```python
from build123d import *

# Parameters (mm, degrees)
SKETCH_R  = 1.25
PAD_DEPTH = 10
FILLET_R  = 1


with BuildPart() as part:
    # Sketch → Pad (new body)
    with BuildSketch(Plane.XY):
        Polygon((-7.5, 7.5), (-1.7, 7.5), (-1.7, 6.4), (-2.85, 6.4), (-2.85, 3.8), (-1.7, 2.802683), (1.7, 2.802683), (2.85, 3.8), (2.85, 6.4), (1.7, 6.4), (1.7, 7.5), (7.5, 7.5), (7.5, 1.7), (6.4, 1.7), (6.4, 2.85), (3.8, 2.85), (2.802683, 1.7), (2.802683, -1.7), (3.8, -2.85), (6.4, -2.85), (6.4, -1.7), (7.5, -1.7), (7.5, -7.5), (1.7, -7.5), (1.7, -6.4), (2.85, -6.4), (2.85, -3.8), (1.7, -2.802683), (-1.7, -2.802683), (-2.85, -3.8), (-2.85, -6.4), (-1.7, -6.4), (-1.7, -7.5), (-7.5, -7.5), (-7.5, -1.7), (-6.4, -1.7), (-6.4, -2.85), (-3.8, -2.85), (-2.802683, -1.7), (-2.802683, 1.7), (-3.8, 2.85), (-6.4, 2.85), (-6.4, 1.7), (-7.5, 1.7), align=None)
        Circle(SKETCH_R, mode=Mode.SUBTRACT)
    extrude(amount=PAD_DEPTH)

    # Fillet
    fillet_edges = [part.edges().sort_by_distance(p)[0] for p in [
        (-7.5, -7.5, 5),
        (7.5, -7.5, 5),
        (7.5, 7.5, 5),
        (-7.5, 7.5, 5),
    ]]
    fillet(fillet_edges, radius=FILLET_R)


solid = part.part
```
For this review, take the finished solid that the model builds, in its own axes (mm). A direction names the side the tool comes from. Round coordinates to 2 decimals unless told otherwise and drop trailing zeros. Loops run counter-clockwise (first coordinate to the right, second up) from the corner with the lowest first, then second, coordinate; pieces in that order, holes last.
Q1. Add section A-A on x = 0. Write out the cut boundary in (y, z).
Result sheet:
outline: (-2.8, 0) - (-1.25, 0) - (-1.25, 10) - (-2.8, 10) - close; (1.25, 0) - (2.8, 0) - (2.8, 10) - (1.25, 10) - close
Q2. Add section C-C on x = -2. Write out the cut boundary in (y, z).
Result sheet:
outline: (-7.5, 0) - (-6.4, 0) - (-6.4, 10) - (-7.5, 10) - close; (-3.06, 0) - (3.06, 0) - (3.06, 10) - (-3.06, 10) - close; (6.4, 0) - (7.5, 0) - (7.5, 10) - (6.4, 10) - close
Q3. Machinability: for faces 4 (the face through (-1.7, 7, 5)), 5 (the face through (-7, 1.7, 5)), 6 (the face through (-1.7, -7, 5)), 7 (the face through (6.4, -2, 5)), 8 (the face through (4, 7.5, 5)), which of the approach directions +Z, -Z, +X, -X, +Y, -Y give a long, thin tool a straight path to every point of the face, cutting with its end or side? Answer none if there is none.
Result sheet:
face 4: +Z, -Z, +Y
face 5: +Z, -Z, -X
face 6: +Z, -Z, -Y
face 7: +Z, -Z
face 8: +Z, -Z, +X, -X, +Y
Q4. Mouldability with a two-part tool opening along Y and no side actions: class faces 1 (the face through (1.7, -7, 5)), 2 (the face through (2.85, -5, 5)), 3 (the face through (0, 2.803, 5)) as +Y half, -Y half, draft (parallel to the pull), parting line (faces both ways), or undercut.
Result sheet:
face 1: draft
face 2: undercut
face 3: +Y half
Q5. Add section D-D on x = 1.5. Write out the cut boundary in (y, z), plus the area to 3 significant figures.
Result sheet:
outline: (-2.8, 0) - (2.8, 0) - (2.8, 10) - (-2.8, 10) - close
area: 56.1 mm2
Q6. Insertion check: pin 1 Ø3 at (x, y) = (0, 4.5) entering from +Z; pin 2 Ø0.5 at (y, z) = (-7, 4) entering from -X. Each pin has a flat end and moves straight along its axis. Give the tip position at first contact, or say it passes through.
Result sheet:
pin 1: passes through
pin 2: stops at x = -7.47
Q7. Add section B-B on y = -4. Write out the cut boundary in (x, z).
Result sheet:
outline: (-7.5, 0) - (-2.85, 0) - (-2.85, 10) - (-7.5, 10) - close; (2.85, 0) - (7.5, 0) - (7.5, 10) - (2.85, 10) - close
Q8. To check wall thickness, follow line 1 along Y through (x, z) = (-5.5, 4.5); line 2 along Y through (x, z) = (0, 2.5); line 3 along X through (y, z) = (-2.75, 2). State the ranges of each line that lie inside material, in increasing order.
Result sheet:
line 1: y = -7.5 to -2.85, 2.85 to 7.5
line 2: y = -2.8 to -1.25, 1.25 to 2.8
line 3: x = -7.5 to -6.4, -3.71 to 3.71, 6.4 to 7.5
